The figure shows three views and two pictorial views of one solid part (mm, origin at its lowest corner). Answer the questions. A direction names the side the tool comes from. Round coordinates to 2 decimals unless told otherwise and drop trailing zeros. Order: outer loops, then holes, each group sorted by start corner. A loop starts at its lowest first (then second) coordinate and runs counter-clockwise, first axis right, second up. Notation, with made-up numbers: (74, 46.5) -> (91, 46.5) arc R24 cw to (91, 74.5) -> close; hole circle Ø6 at (6, 84.25). An arc over 180 degrees is marked (long way). One line per item, written item: value. Start each with the question number.
1. Section C-C (z = 6) is taken. Give the vertices of the cut face in (x, y).
2. Section D-D (x = 14.5) is taken. Give the vertices of the cut face in (y, z).
3. Section A-A (x = 18.5) is taken. Give the vertices of the cut face in (y, z).
4. Consider line 1 (Y direction, x = 5.5, z = 25.5); line 2 (Y direction, x = 24.5, z = 2); line 3 (X direction, y = 4.5, z = 32). Determine where each line is inside the solid, lowest interval first.
5. Flat-ended cylindrical pins translate along their axes: pin 1 Ø3 at (y, z) = (51.5, 12.5) entering from -X; pin 2 Ø5 at (x, y) = (32.5, 40.5) entering from -Z; pin 3 Ø5 at (x, y) = (28.5, 40) entering from -Z. Find the tip coordinate at first contact, or state that the pin passes through.
6. For the marked faces 1, 2 and 3, determine the directions among +Z, -Z, +X, -X, +Y, -Y from which every point of the face is accessible in a straight line to the end or side of a thin tool.
7. Section B-B (y = 57) is taken. Give the vertices of the cut face in (x, z), then the cut area to 3 significant figures.
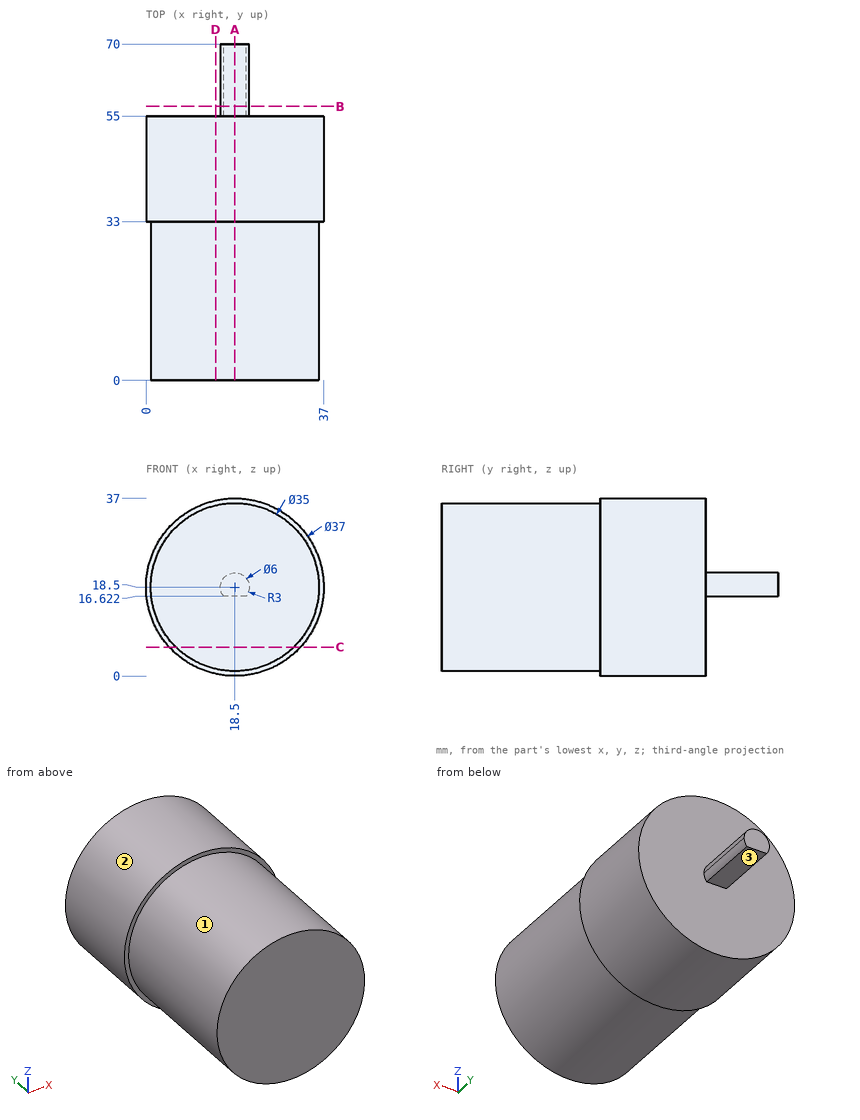
Answer:
1. outline: (4.86, 33) -> (6.25, 33) -> (6.25, 0) -> (30.75, 0) -> (30.75, 33) -> (32.14, 33) -> (32.14, 55) -> (4.86, 55) -> close
2. outline: (0, 1.46) -> (33, 1.46) -> (33, 0.44) -> (55, 0.44) -> (55, 36.56) -> (33, 36.56) -> (33, 35.54) -> (0, 35.54) -> close
3. outline: (0, 1) -> (33, 1) -> (33, 0) -> (55, 0) -> (55, 16.62) -> (70, 16.62) -> (70, 21.5) -> (55, 21.5) -> (55, 37) -> (33, 37) -> (33, 36) -> (0, 36) -> close
4. line 1: 0 to 55
4. line 2: 33 to 55
4. line 3: 7.36 to 29.64
5. pin 1: x = 0.56
5. pin 2: z = 4.01
5. pin 3: z = 1.59
6. face 1: -Y
6. face 2: +Y, -Y
6. face 3: -Z, +X, -X, +Y
7. outline: (16.16, 16.62) -> (20.84, 16.62) arc R3 ccw (long way) to start
7. area: 24.6 mm^2
